from build123d import *

# Parameters (mm, degrees)
SKETCH3_W                                      = 180
SKETCH3_H                                      = 90
BOSS_EXTRUDE3_DEPTH                            = 3
SKETCH4_W                                      = 8.5
SKETCH4_H                                      = 61.5
CUT_EXTRUDE1_DEPTH                             = 3
CSK_FOR_M5_FLAT_HEAD_MACHINE_SCREW1_AT_2_COUNT = 2
CSK_FOR_M5_FLAT_HEAD_MACHINE_SCREW1_AT_2_PITCH = 167.524625056
CSK_FOR_M5_FLAT_HEAD_MACHINE_SCREW1_AT_3_COUNT = 2
CSK_FOR_M5_FLAT_HEAD_MACHINE_SCREW1_AT_3_PITCH = 71.5
CSK_FOR_M5_FLAT_HEAD_MACHINE_SCREW1_AT_4_COUNT = 2
CSK_FOR_M5_FLAT_HEAD_MACHINE_SCREW1_AT_4_PITCH = 151.5
CSK_SLOT_FOR_M5_FLAT_HEAD_MACHINE_SCREW1_DEPTH = 3
SKETCH12_W                                     = 9.5
SKETCH12_H                                     = 10
BOSS_EXTRUDE4_DEPTH                            = 10
CSK_FOR_M4_SFHCS1_D                            = 4.5
CSK_FOR_M4_SFHCS1_DEPTH                        = 10
CSK_FOR_M4_SFHCS1_CSINK_D                      = 8.96
CSK_FOR_M4_SFHCS1_CSINK_ANGLE                  = 90
M4X0_7_TAPPED_HOLE1_D                          = 3.3


with BuildPart() as part:
    # Sketch3 → Boss-Extrude3 (new body)
    with BuildSketch(Plane.XY):
        Rectangle(SKETCH3_W, SKETCH3_H)
    extrude(amount=BOSS_EXTRUDE3_DEPTH)

    # Sketch4 → Cut-Extrude1 (cut)
    with BuildSketch(Plane.XY.offset(3)):
        with BuildLine():
            Line((-4.25, -30.75), (-4.25, 30.75))
            ThreePointArc((-4.25, 30.75), (-7.785533906, 32.214466094), (-9.25, 35.75))
            Line((-9.25, 35.75), (-70.75, 35.75))
            ThreePointArc((-70.75, 35.75), (-72.214466094, 32.214466094), (-75.75, 30.75))
            Line((-75.75, 30.75), (-75.75, -30.75))
            ThreePointArc((-75.75, -30.75), (-72.214466094, -32.214466094), (-70.75, -35.75))
            Line((-70.75, -35.75), (-9.25, -35.75))
            ThreePointArc((-9.25, -35.75), (-7.785533906, -32.214466094), (-4.25, -30.75))
        make_face()
        Rectangle(SKETCH4_W, SKETCH4_H)
        with BuildLine():
            ThreePointArc((9.25, 35.75), (7.785533906, 32.214466094), (4.25, 30.75))
            Line((4.25, 30.75), (4.25, -30.75))
            ThreePointArc((4.25, -30.75), (7.785533906, -32.214466094), (9.25, -35.75))
            Line((9.25, -35.75), (70.75, -35.75))
            ThreePointArc((70.75, -35.75), (72.214466094, -32.214466094), (75.75, -30.75))
            Line((75.75, -30.75), (75.75, 30.75))
            ThreePointArc((75.75, 30.75), (72.214466094, 32.214466094), (70.75, 35.75))
            Line((70.75, 35.75), (9.25, 35.75))
        make_face()
    extrude(amount=-CUT_EXTRUDE1_DEPTH, mode=Mode.SUBTRACT)

    # Sketch8 → CSK for M5 Flat Head Machine Screw1 (revolve, cut)
    with BuildSketch(Plane(origin=(-75.75, 35.75, 3), x_dir=(0, -1, 0), z_dir=(1, 0, 0))):
        Polygon((0, 0), (0, 3), (2.55, 3), (2.55, 0.85), (3.4, 0), align=None)
    csk_for_m5_flat_head_machine_screw1 = revolve(axis=Axis((-75.75, 35.75, 9.35), (0, 0, -1)), mode=Mode.SUBTRACT)

    # CSK for M5 Flat Head Machine Screw1 at 2: CSK for M5 Flat Head Machine Screw1 ×2
    with Locations(*[Vector(0.9043446594777974, -0.4268029251000826, 0) * (i * CSK_FOR_M5_FLAT_HEAD_MACHINE_SCREW1_AT_2_PITCH) for i in range(1, CSK_FOR_M5_FLAT_HEAD_MACHINE_SCREW1_AT_2_COUNT)]):
        add(csk_for_m5_flat_head_machine_screw1, mode=Mode.SUBTRACT)

    # CSK for M5 Flat Head Machine Screw1 at 3: CSK for M5 Flat Head Machine Screw1 ×2
    with Locations(*[(0, -i * CSK_FOR_M5_FLAT_HEAD_MACHINE_SCREW1_AT_3_PITCH, 0) for i in range(1, CSK_FOR_M5_FLAT_HEAD_MACHINE_SCREW1_AT_3_COUNT)]):
        add(csk_for_m5_flat_head_machine_screw1, mode=Mode.SUBTRACT)

    # CSK for M5 Flat Head Machine Screw1 at 4: CSK for M5 Flat Head Machine Screw1 ×2
    with Locations(*[(i * CSK_FOR_M5_FLAT_HEAD_MACHINE_SCREW1_AT_4_PITCH, 0, 0) for i in range(1, CSK_FOR_M5_FLAT_HEAD_MACHINE_SCREW1_AT_4_COUNT)]):
        add(csk_for_m5_flat_head_machine_screw1, mode=Mode.SUBTRACT)

    # CSK SLOT for M5 Flat Head Machine Screw1: read off the stored shape, not the designer's step
    # CSK SLOT for M5 Flat Head Machine Sc 2 → CSK SLOT for M5 Flat Head Machine Screw1 (cut)
    with BuildSketch(Plane.XY):
        with BuildLine():
            Line((-4.25, 33.2), (4.25, 33.2))
            ThreePointArc((4.25, 33.2), (6.8, 35.75), (4.25, 38.3))
            Line((4.25, 38.3), (-4.25, 38.3))
            ThreePointArc((-4.25, 38.3), (-6.8, 35.75), (-4.25, 33.2))
        make_face()
        with BuildLine():
            Line((-4.25, -38.3), (4.25, -38.3))
            ThreePointArc((4.25, -38.3), (6.8, -35.75), (4.25, -33.2))
            Line((4.25, -33.2), (-4.25, -33.2))
            ThreePointArc((-4.25, -33.2), (-6.8, -35.75), (-4.25, -38.3))
        make_face()
    extrude(amount=CSK_SLOT_FOR_M5_FLAT_HEAD_MACHINE_SCREW1_DEPTH, mode=Mode.SUBTRACT)

    # CSK SLOT for M5 Flat Head Machine Sc 3: loft between two sections, ruled curve by curve
    csk_slot_for_m5_flat_head_machine_sc_3_from = [
        Edge.make_three_point_arc((4.25, 33.2, 2.15), (6.053122292, 33.946877708, 2.15), (6.8, 35.75, 2.15)),
        Edge.make_three_point_arc((6.8, 35.75, 2.15), (6.053122292, 37.553122292, 2.15), (4.25, 38.3, 2.15)),
        Edge.make_three_point_arc((-4.25, 38.3, 2.15), (-6.053122292, 37.553122292, 2.15), (-6.8, 35.75, 2.15)),
        Edge.make_three_point_arc((-6.8, 35.75, 2.15), (-6.053122292, 33.946877708, 2.15), (-4.25, 33.2, 2.15)),
        Edge.make_line((4.25, 38.3, 2.15), (-4.25, 38.3, 2.15)),
        Edge.make_line((4.25, 33.2, 2.15), (-4.25, 33.2, 2.15)),
    ]
    csk_slot_for_m5_flat_head_machine_sc_3_to = [
        Edge.make_three_point_arc((4.25, 32.35, 3), (6.654163056, 33.345836944, 3), (7.65, 35.75, 3)),
        Edge.make_three_point_arc((7.65, 35.75, 3), (6.654163056, 38.154163056, 3), (4.25, 39.15, 3)),
        Edge.make_three_point_arc((-4.25, 39.15, 3), (-6.654163056, 38.154163056, 3), (-7.65, 35.75, 3)),
        Edge.make_three_point_arc((-7.65, 35.75, 3), (-6.654163056, 33.345836944, 3), (-4.25, 32.35, 3)),
        Edge.make_line((4.25, 39.15, 3), (-4.25, 39.15, 3)),
        Edge.make_line((4.25, 32.35, 3), (-4.25, 32.35, 3)),
    ]
    csk_slot_for_m5_flat_head_machine_sc_3 = Solid(Shell([*[Face.make_surface_from_curves(csk_slot_for_m5_flat_head_machine_sc_3_from[k], csk_slot_for_m5_flat_head_machine_sc_3_to[k]) for k in range(6)], Face(Wire(csk_slot_for_m5_flat_head_machine_sc_3_from)), Face(Wire(csk_slot_for_m5_flat_head_machine_sc_3_to))]))
    add(csk_slot_for_m5_flat_head_machine_sc_3, mode=Mode.SUBTRACT)

    # CSK SLOT for M5 Flat Head Machine Sc 4: loft between two sections, ruled curve by curve
    csk_slot_for_m5_flat_head_machine_sc_4_from = [
        Edge.make_three_point_arc((4.25, -38.3, 2.15), (6.053122292, -37.553122292, 2.15), (6.8, -35.75, 2.15)),
        Edge.make_three_point_arc((6.8, -35.75, 2.15), (6.053122292, -33.946877708, 2.15), (4.25, -33.2, 2.15)),
        Edge.make_three_point_arc((-4.25, -33.2, 2.15), (-6.053122292, -33.946877708, 2.15), (-6.8, -35.75, 2.15)),
        Edge.make_three_point_arc((-6.8, -35.75, 2.15), (-6.053122292, -37.553122292, 2.15), (-4.25, -38.3, 2.15)),
        Edge.make_line((4.25, -33.2, 2.15), (-4.25, -33.2, 2.15)),
        Edge.make_line((4.25, -38.3, 2.15), (-4.25, -38.3, 2.15)),
    ]
    csk_slot_for_m5_flat_head_machine_sc_4_to = [
        Edge.make_three_point_arc((4.25, -39.15, 3), (6.654163056, -38.154163056, 3), (7.65, -35.75, 3)),
        Edge.make_three_point_arc((7.65, -35.75, 3), (6.654163056, -33.345836944, 3), (4.25, -32.35, 3)),
        Edge.make_three_point_arc((-4.25, -32.35, 3), (-6.654163056, -33.345836944, 3), (-7.65, -35.75, 3)),
        Edge.make_three_point_arc((-7.65, -35.75, 3), (-6.654163056, -38.154163056, 3), (-4.25, -39.15, 3)),
        Edge.make_line((4.25, -32.35, 3), (-4.25, -32.35, 3)),
        Edge.make_line((4.25, -39.15, 3), (-4.25, -39.15, 3)),
    ]
    csk_slot_for_m5_flat_head_machine_sc_4 = Solid(Shell([*[Face.make_surface_from_curves(csk_slot_for_m5_flat_head_machine_sc_4_from[k], csk_slot_for_m5_flat_head_machine_sc_4_to[k]) for k in range(6)], Face(Wire(csk_slot_for_m5_flat_head_machine_sc_4_from)), Face(Wire(csk_slot_for_m5_flat_head_machine_sc_4_to))]))
    add(csk_slot_for_m5_flat_head_machine_sc_4, mode=Mode.SUBTRACT)

    # Sketch12 → Boss-Extrude4 (add)
    with BuildSketch(Plane(origin=(0, 0, 0), x_dir=(-1, 0, 0), z_dir=(0, 0, -1))):
        with Locations((-85.25, 40)):
            Rectangle(SKETCH12_W, SKETCH12_H)
        with Locations((-85.25, -40)):
            Rectangle(SKETCH12_W, SKETCH12_H)
    boss_extrude4 = extrude(amount=BOSS_EXTRUDE4_DEPTH)

    # CSK for M4 SFHCS1
    with Locations(Plane(origin=(0, -35, 0), x_dir=(1, 0, 0), z_dir=(0, 1, 0))):
        with Locations((85.162636167, 5)):
            csk_for_m4_sfhcs1 = CounterSinkHole(CSK_FOR_M4_SFHCS1_D / 2, CSK_FOR_M4_SFHCS1_CSINK_D / 2, depth=CSK_FOR_M4_SFHCS1_DEPTH, counter_sink_angle=CSK_FOR_M4_SFHCS1_CSINK_ANGLE)

    # M4x0.7 Tapped Hole1 (through all)
    with Locations(Plane(origin=(0, 45, 0), x_dir=(1, 0, 0), z_dir=(0, 1, 0))):
        with Locations((85.25, 5)):
            m4x0_7_tapped_hole1 = Hole(M4X0_7_TAPPED_HOLE1_D / 2)

    # Mirror1: Boss-Extrude4, CSK for M4 SFHCS1, M4x0.7 Tapped Hole1 across plane
    add(boss_extrude4.mirror(Plane(origin=(0, 0, 0), x_dir=(0, 0, 1), z_dir=(1, 0, 0))))
    add(csk_for_m4_sfhcs1.mirror(Plane(origin=(0, 0, 0), x_dir=(0, 0, 1), z_dir=(1, 0, 0))), mode=Mode.SUBTRACT)
    add(m4x0_7_tapped_hole1.mirror(Plane(origin=(0, 0, 0), x_dir=(0, 0, 1), z_dir=(1, 0, 0))), mode=Mode.SUBTRACT)


solid = part.part
Geometry: final body of the model. Coordinates: model frame, mm. A direction names the side the tool comes from. Give positions to 0.01 mm unless a question says otherwise; leave off trailing zeros. Order: outer loops, then holes, each group sorted by start corner. A loop starts at its lowest first (then second) coordinate and runs counter-clockwise, first axis right, second up. Notation, with made-up numbers: (81.25, 69.25) - (108.25, 69.25) arc R29 ccw to (108.25, 90.25) - close; hole circle Ø3 at (32.25, 15). An arc over 180 degrees is marked (long way). Use CSV: the item, a comma, the result in double quotes.
1. Material intervals for line 1 along Y through (x, z) = (15.5, 1.25); line 2 along Z through (x, y) = (85, 39); line 3 along Z through (x, y) = (77.5, 7), sorted ascending. Write a range as from..to.
Answers below:
line 1,"-45..-35.75, 35.75..45"
line 2,"-10..-6.63, -3.37..3"
line 3,"0..3"
2. Mould query, pull axis X, two halves, no side actions, for faces 1 (the face through (83, 35, -5)), 2 (the face through (-86.9, 39.93, -5.07)), 3 (the face through (90, -1, 1)). Classes: +X half, -X half, draft (parallel to the pull), parting line (faces both ways), or undercut.
Answers below:
face 1,"draft"
face 2,"undercut"
face 3,"+X half"
3. Section query A-A (x = 12). Output: boundary loops of the cut face in (y, z).
Answers below:
outline,"(-45, 0) - (-35.75, 0) - (-35.75, 3) - (-45, 3) - close; (35.75, 0) - (45, 0) - (45, 3) - (35.75, 3) - close"
4. Access query for faces 4 (the face through (80.5, -40, -5)), 5 (the face through (7.82, 32.25, 1.52)), 6 (the face through (-87.41, -41.17, -5.1)), 7 (the face through (-88.44, -35, -8.31)). Directions: +Z, -Z, +X, -X, +Y, -Y. A direction counts if a zero-diameter tool reaches every point of the face in a straight line with its end or side. Return the directions, or none.
Answers below:
face 4,"-Z, +Y, -Y"
face 5,"+Z, -Z"
face 6,"-Y"
face 7,"-Z, +X, -X"
5. Section query B-B (y = -15). Output: boundary loops of the cut face in (x, z), plus the area to 3 significant figures.
Answers below:
outline,"(-90, 0) - (-75.75, 0) - (-75.75, 3) - (-90, 3) - close; (75.75, 0) - (90, 0) - (90, 3) - (75.75, 3) - close"
area,"85.5 mm2"
6. Contact query for flat-ended pins moving along their axis: pin 1 (2 mm diameter, centred on x = 85.25, z = -5, fed in from +Y); pin 2 (6 mm diameter, centred on x = 85.16, z = -5, fed in from +Y). Output: stop coordinate, or through.
Answers below:
pin 1,"through"
pin 2,"y = 45"
7. Section query C-C (z = -5). Give the number of separate pieces and of enclosed holes in the cut face, plus the area to 3 significant figures.
Answers below:
separate pieces,"8"
enclosed holes,"0"
area,"214 mm2"
